Geometry: final body of the model. Coordinates: model frame, mm. Face numbers are marked on the shaded views. A direction names the side the tool comes from. Round coordinates to 2 decimals unless told otherwise and drop trailing zeros. Loops run counter-clockwise (first coordinate to the right, second up) from the corner with the lowest first, then second, coordinate; pieces in that order, holes last. Notation, with made-up numbers: (19, 20.5) -> (78, 20.5) arc R20 cw to (78, 32.5) -> close; hole circle Ø5 at (14.5, -16). An arc over 180 degrees is marked (long way). Answer in a Markdown table with one row per item.
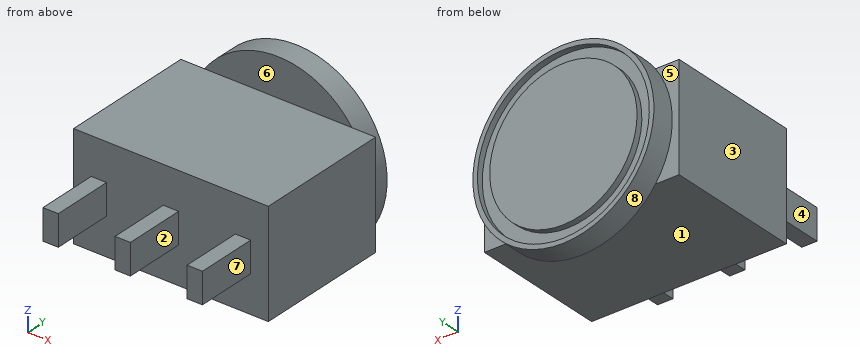
```python
from build123d import *

# Parameters (mm, degrees)
BOSS_EXTRUDE1_DEPTH      = 3.43
BOSS_EXTRUDE1_DEPTH_BACK = 3.43
SKETCH1_W                = 12.7
SKETCH1_H                = 8.89
BOSS_EXTRUDE2_DEPTH      = 1
BOSS_EXTRUDE2_DEPTH_BACK = 1
SKETCH2_W                = 1
SKETCH2_H                = 4


with BuildPart() as part:
    # Sketch1 → Boss-Extrude1 (new, two sides: drawn at the far end of the back side and taken through both)
    with BuildSketch(Plane.XY.offset(-BOSS_EXTRUDE1_DEPTH_BACK)):
        with Locations((0, -4.445)):
            Rectangle(SKETCH1_W, SKETCH1_H)
    extrude(amount=BOSS_EXTRUDE1_DEPTH + BOSS_EXTRUDE1_DEPTH_BACK)

    # Sketch2 → Boss-Extrude2 (add, two sides: drawn at the far end of the back side and taken through both)
    with BuildSketch(Plane.XY.offset(-BOSS_EXTRUDE2_DEPTH_BACK)):
        with Locations((-4.7, -10.89)):
            Rectangle(SKETCH2_W, SKETCH2_H)
        with Locations((0, -10.89)):
            Rectangle(SKETCH2_W, SKETCH2_H)
        with Locations((4.7, -10.89)):
            Rectangle(SKETCH2_W, SKETCH2_H)
    extrude(amount=BOSS_EXTRUDE2_DEPTH + BOSS_EXTRUDE2_DEPTH_BACK)

    # Sketch3 → Revolve1 (revolve)
    with BuildSketch(Plane.XY, mode=Mode.PRIVATE) as revolve1_sk:
        Polygon((0, 0), (0, 1.524), (4.805, 1.524), (4.805, 1.124), (5.605, 1.124), (5.605, 1.524), (5.905, 1.524), (5.905, 0), align=None)
    revolve(revolve1_sk.sketch.rotate(Axis((0, 0, 0), (0, 1, 0)), 90), axis=Axis((0, 0, 0), (0, 1, 0)))


solid = part.part
```
Item 1: Cut plane A-A (x = 0). Output: boundary loops of the cut face in (y, z) (3 decimals), then the cut area to 3 significant figures.
Answer:
| item | result |
|---|---|
| outline | (-12.89, -1) -> (-8.89, -1) -> (-8.89, -3.43) -> (0, -3.43) -> (0, -5.905) -> (1.524, -5.905) -> (1.524, -5.605) -> (1.124, -5.605) -> (1.124, -4.805) -> (1.524, -4.805) -> (1.524, 4.805) -> (1.124, 4.805) -> (1.124, 5.605) -> (1.524, 5.605) -> (1.524, 5.905) -> (0, 5.905) -> (0, 3.43) -> (-8.89, 3.43) -> (-8.89, 1) -> (-12.89, 1) -> close |
| area | 86.3 mm² |
Item 2: Cut plane C-C (y = -7.5). Output: boundary loops of the cut face in (x, z).
Answer:
| item | result |
|---|---|
| outline | (-6.35, -3.43) -> (6.35, -3.43) -> (6.35, 3.43) -> (-6.35, 3.43) -> close |
Item 3: Line query: probe 1 along X at (y, z) = (1.25, 0) (3 decimals); probe 2 along Y at (x, z) = (4.5, 3.75); probe 3 along Z at (x, y) = (-1.25, -4.5). Output: solid intervals per line, ascending. Write a range as [from, to].
Answer:
| item | result |
|---|---|
| probe 1 | x = [-5.905, -5.605], [-4.805, 4.805], [5.605, 5.905] |
| probe 2 | y = [0, 1.52] |
| probe 3 | z = [-3.43, 3.43] |
Item 4: Reachability of the marked faces 4, 5, 6, 7 and 8 from +Z, -Z, +X, -X, +Y, -Y: full face, straight path, thin tool, end or side. Return the list, or none.
Answer:
| item | result |
|---|---|
| face 4 | +Z, -Z, -X, -Y |
| face 5 | -X, +Y |
| face 6 | +Z, +X, -X, -Y |
| face 7 | +Z, -Z, +X, -Y |
| face 8 | +Y |
Item 5: Draft query along X for the marked faces 1, 2 and 3. Return one class per face: pulls with the +X half, pulls with the -X half, needs draft (parallel to the pull), parting line crosses it, or undercut.
Answer:
| item | result |
|---|---|
| face 1 | needs draft |
| face 2 | undercut |
| face 3 | pulls with the -X half |
Item 6: Cut plane B-B (z = 0). Output: boundary loops of the cut face in (x, y) (3 decimals).
Answer:
| item | result |
|---|---|
| outline | (-6.35, -8.89) -> (-5.2, -8.89) -> (-5.2, -12.89) -> (-4.2, -12.89) -> (-4.2, -8.89) -> (-0.5, -8.89) -> (-0.5, -12.89) -> (0.5, -12.89) -> (0.5, -8.89) -> (4.2, -8.89) -> (4.2, -12.89) -> (5.2, -12.89) -> (5.2, -8.89) -> (6.35, -8.89) -> (6.35, 0) -> (5.905, 0) -> (5.905, 1.524) -> (5.605, 1.524) -> (5.605, 1.124) -> (4.805, 1.124) -> (4.805, 1.524) -> (-4.805, 1.524) -> (-4.805, 1.124) -> (-5.605, 1.124) -> (-5.605, 1.524) -> (-5.905, 1.524) -> (-5.905, 0) -> (-6.35, 0) -> close |
Item 7: Pin query (flat end, axial travel): pin 1 Ø2 at (x, z) = (2.5, -1) entering from -Y; pin 2 Ø0.8 at (x, y) = (4.5, -11) entering from -Z; pin 3 Ø3 at (x, y) = (2.5, -3.5) entering from +Z. Return the tip coordinate at first contact, or that it passes through.
Answer:
| item | result |
|---|---|
| pin 1 | stops at y = -8.89 |
| pin 2 | stops at z = -1 |
| pin 3 | stops at z = 3.43 |
Item 8: Cut plane D-D (z = 2). Output: boundary loops of the cut face in (x, y).
Answer:
| item | result |
|---|---|
| outline | (-6.35, -8.89) -> (6.35, -8.89) -> (6.35, 0) -> (5.56, 0) -> (5.56, 1.52) -> (5.24, 1.52) -> (5.24, 1.12) -> (4.37, 1.12) -> (4.37, 1.52) -> (-4.37, 1.52) -> (-4.37, 1.12) -> (-5.24, 1.12) -> (-5.24, 1.52) -> (-5.56, 1.52) -> (-5.56, 0) -> (-6.35, 0) -> close |
